from build123d import *

# Parameters (mm, degrees)
EXTRUDE_1_DEPTH     = 16
FILLET_1_R          = 8
FILLET_2_R          = 3
SKETCH_2_R          = 4.25
CUT_EXTRUDE_1_DEPTH = 48.201694885


with BuildPart() as part:
    # Эскиз1 → Бобышка-Вытянуть1 (new body)
    with BuildSketch(Plane(origin=(0, 0, 0), x_dir=(1, 0, 0), z_dir=(0, 1, 0))):
        Polygon((0, 18), (0, -18), (26, -18), (26, -13), (5, -13), (5, 13), (26, 13), (26, 18), align=None)
    extrude(amount=EXTRUDE_1_DEPTH)

    # Скругление1
    fillet_1_edges = [part.edges().sort_by_distance(p)[0] for p in [
        (26, 0, -15.5),
        (26, 16, -15.5),
        (26, 0, 15.5),
        (26, 16, 15.5),
    ]]
    fillet(fillet_1_edges, radius=FILLET_1_R - 0.0001)  # a hair under: the kernel refuses the full size

    # Скругление2
    fillet_2_edges = [part.edges().sort_by_distance(p)[0] for p in [
        (0, 8, 18),
        (0, 8, -18),
    ]]
    fillet(fillet_2_edges, radius=FILLET_2_R)

    # Эскиз2 → Вырез-Вытянуть1 (cut, through all)
    with BuildSketch(Plane.XY.offset(18)):
        with Locations((18, 8)):
            Circle(SKETCH_2_R)
    extrude(amount=-CUT_EXTRUDE_1_DEPTH, mode=Mode.SUBTRACT)


solid = part.part
Verification items for the finished model (mm, model axes). A direction names the side the tool comes from. Coordinates: 2 decimals unless noted, no trailing zeros. Order: outer loops, then holes, each group sorted by start corner. A loop starts at its lowest first (then second) coordinate and runs counter-clockwise, first axis right, second up.
1. Sectioned sample at C-C, the plane y = 13.75. Record the cut outline in (x, z).
Results found:
outline: (0, -15) arc R3 ccw to (3, -18) - (23.56, -18) - (23.56, -13) - (5, -13) - (5, 13) - (23.56, 13) - (23.56, 18) - (3, 18) arc R3 ccw to (0, 15) - close
2. Go/stop test with a flat-tipped pin: pin 1 Ø5 at (x, y) = (18, 8) entering from +Z. Record where the tip stops, or that it passes through.
Results found:
pin 1: passes through
3. Release check for a two-part mould opening along Z. For faces 1 (the face through (3, 16, 0)), 2 (the face through (5, 8, 0)), 3 (the face through (12, 8, -18)) record: +Z half, -Z half, draft (parallel to the pull), parting line (faces both ways), or undercut.
Results found:
face 1: draft
face 2: undercut
face 3: -Z half
4. Sectioned sample at A-A, the plane x = 6.5. Record the cut outline in (y, z).
Results found:
outline: (0, -18) - (16, -18) - (16, -13) - (0, -13) - close; (0, 13) - (16, 13) - (16, 18) - (0, 18) - close
5. Set-up check for faces 4 (the face through (13, 8, 13)), 5 (the face through (23.719, 2.406, 15.465)): record each of +Z, -Z, +X, -X, +Y, -Y from which the full face is reachable in a straight line by a thin tool's end or side.
Results found:
face 4: +X, +Y, -Y
face 5: +Z, -Z, +X, -Y
6. Scan lines: line 1 (Y direction, x = 18, z = 14.6); line 2 (Z direction, x = 17.75, y = 13.25); line 3 (X direction, y = 4.5, z = -11). Record each from-to range of solid material in increasing order.
Results found:
line 1: y = 0 to 3.75, 12.25 to 16
line 2: z = -18 to -13, 13 to 18
line 3: x = 0 to 5
7. Sectioned sample at B-B, the plane y = 10.75. Record the cut outline in (x, z), and give its area (3 significant figures).
Results found:
outline: (0, -15) arc R3 ccw to (3, -18) - (14.76, -18) - (14.76, -13) - (5, -13) - (5, 13) - (14.76, 13) - (14.76, 18) - (3, 18) arc R3 ccw to (0, 15) - close; (21.24, -18) - (25.51, -18) - (25.51, -13) - (21.24, -13) - close; (21.24, 13) - (25.51, 13) - (25.51, 18) - (21.24, 18) - close
area: 316 mm2
8. Sectioned sample at D-D, the plane z = 5.5. Record the cut outline in (x, y), and give its area (3 significant figures).
Results found:
outline: (0, 0) - (5, 0) - (5, 16) - (0, 16) - close
area: 80.0 mm2
